Can you work these out from the model? Positions are in its coordinate system, mm. Give positions to 0.01 mm unless a question says otherwise; leave off trailing zeros. Loops run counter-clockwise (first coordinate to the right, second up) from the corner with the lowest first, then second, coordinate; pieces in that order, holes last.
from build123d import *

# Parameters (mm, degrees)
F0_R     = 1.6
F1_DEPTH = 3.2
F2_R     = 1.6
F3_DEPTH = 6


with BuildPart() as f1:
    # F0 (on Front) → F1 (new body)
    with BuildSketch(Plane.XZ):
        Polygon((83.125, -21.650635), (103.125, 12.990381), (-66.875, 12.990381), (-86.875, -21.650635), align=None)
        with Locations((-69.554492, -11.650635)):
            Circle(F0_R, mode=Mode.SUBTRACT)
        with Locations((85.804492, 2.990381)):
            Circle(F0_R, mode=Mode.SUBTRACT)
    extrude(amount=F1_DEPTH)

    # F2 (on face) → F3 (cut)
    with BuildSketch(Plane.XZ.offset(3.2)):
        with Locations((-8.611966, -11.650635)):
            Circle(F2_R)
    extrude(amount=-F3_DEPTH, mode=Mode.SUBTRACT)


solid = f1.part
(1) Suppose I cut it at B-B on z = -3.5. List the corners of the cut face in (x, y) for me, plus the area to 3 significant figures.
Returned:
outline: (-76.4, -3.2) - (93.6, -3.2) - (93.6, 0) - (-76.4, 0) - close
area: 544 mm2
(2) Thinking about a two-plate mould opening in X: for faces 1 (the flat face through (-76.735, -1.578, -4.088)), 2 (the cylindrical face through (87.282, -1.578, 2.378)), 3 (the flat face through (92.985, -1.578, -4.573)), 4 (the flat face through (7, -3.2, -4)), which applies, pulls with the +X half, pulls with the -X half, needs draft (parallel to the pull), parting line crosses it, or undercut?
Returned:
face 1: pulls with the -X half
face 2: undercut
face 3: pulls with the +X half
face 4: needs draft
(3) Please list where these lines run through material, in increasing order: probe 1 along X at (y, z) = (-0.5, -13); probe 2 along X at (y, z) = (-2.45, 3); probe 3 along X at (y, z) = (-2, -5).
Returned:
probe 1: x = -81.88 to -70.41, -68.69 to -9.47, -7.75 to 88.12
probe 2: x = -72.64 to 84.2, 87.4 to 97.36
probe 3: x = -77.26 to 92.74
(4) Suppose I cut it at A-A on y = -2.55. List the corners of the cut face in (x, z) for me (1 decimal).
Returned:
outline: (-86.9, -21.7) - (83.1, -21.7) - (103.1, 13) - (-66.9, 13) - close; hole circle Ø3.2 at (-69.6, -11.7); hole circle Ø3.2 at (-8.6, -11.7); hole circle Ø3.2 at (85.8, 3)
(5) Will this pin go through, and if not, where does the flat tip stop? P1, Ø2.5, axis at x = -8.61, z = -11.65, coming from the -Y side.
Returned:
P1: passes through
